Input: part model. Units: mm. Frame: model coordinates. Round coordinates to 2 decimals unless told otherwise and drop trailing zeros. Write each loop counter-clockwise with the first axis right and the second up, starting at its lowest first coordinate (ties: lowest second). Pieces come first, ordered by that corner, then holes. Notation, with made-up numbers: (11, 0.25) - (32, 0.25) arc R14 cw to (32, 9.25) - close; hole circle Ø8 at (-26.5, -7). An arc over 180 degrees is marked (long way). Use one line per item in the form item = value.
```python
from build123d import *

# Parameters (mm, degrees)
CHAMFER1_SIZE      = 0.25
CUT_EXTRUDE1_DEPTH = 0.5
FILLET7_R          = 0.5


with BuildPart() as part:
    # Sketch1 → Revolve1 (revolve)
    with BuildSketch(Plane(origin=(0, 0, 0), x_dir=(0, 0, -1), z_dir=(1, 0, 0))):
        Polygon((9.5, 0), (9.5, 1.5), (1.5, 1.5), (1.5, 2.5), (0, 2.5), (0, 0), align=None)
    revolve(axis=Axis((0, 0, 0), (0, 0, -1)))

    # Chamfer1
    chamfer1_edges = [part.edges().sort_by_distance(p)[0] for p in [
        (0, -1.5, -9.5),
    ]]
    chamfer(chamfer1_edges, length=CHAMFER1_SIZE)

    # Sketch2 → Cut-Extrude1 (cut)
    with BuildSketch(Plane.XY):
        with BuildLine():
            Line((-0.15, 2.495495943), (-0.15, 0.15))
            Line((-0.15, 0.15), (-2.495495943, 0.15))
            ThreePointArc((-2.495495943, 0.15), (-2.5, 0), (-2.495495943, -0.15))
            Line((-2.495495943, -0.15), (-0.15, -0.15))
            Line((-0.15, -0.15), (-0.15, -2.495495943))
            ThreePointArc((-0.15, -2.495495943), (0, -2.5), (0.15, -2.495495943))
            Line((0.15, -2.495495943), (0.15, -0.15))
            Line((0.15, -0.15), (2.495495943, -0.15))
            ThreePointArc((2.495495943, -0.15), (2.5, 0), (2.495495943, 0.15))
            Line((2.495495943, 0.15), (0.15, 0.15))
            Line((0.15, 0.15), (0.15, 2.495495943))
            ThreePointArc((0.15, 2.495495943), (0, 2.5), (-0.15, 2.495495943))
        make_face()
    extrude(amount=-CUT_EXTRUDE1_DEPTH, mode=Mode.SUBTRACT)

    # Fillet7
    fillet7_edges = [part.edges().sort_by_distance(p)[0] for p in [
        (-1.767766953, -1.767766953, 0),
        (1.767766953, -1.767766953, 0),
        (1.767766953, 1.767766953, 0),
        (-1.767766953, 1.767766953, 0),
    ]]
    fillet(fillet7_edges, radius=FILLET7_R)


solid = part.part
```
(1) Cut plane C-C on z = -2. Output: boundary loops of the cut face in (x, y).
Derived:
outline = circle Ø3 at (0, 0)
(2) Draft query along X for faces 1 (the face through (0, 0, -0.5)), 2 (the face through (0.07, -1.5, -5.32)), 3 (the face through (0, -2, -1.5)). Return one class per face: released by +X, released by -X, zero draft, split by the parting line, or undercut.
Derived:
face_1 = undercut
face_2 = split by the parting line
face_3 = zero draft
(3) First-contact query: pin 1 Ø2.5 at (x, y) = (1, -1) entering from -Z; pin 2 Ø1.5 at (x, z) = (1.5, -6) entering from -Y. Flat tips, straight axial feed; report the tip coordinate or a pass-through.
Derived:
pin_1 = -9.5
pin_2 = -1.3
(4) Material intervals for L1, parallel to Z at x = 0.8, y = 1.55; L2, parallel to Y at x = 1.1, z = -3.5; L3, parallel to X at y = 1.05, z = -3.75, sorted ascending.
Derived:
L1 = -1.5 to 0
L2 = -1.02 to 1.02
L3 = -1.07 to 1.07
(5) Cut plane A-A on x = 0. Output: boundary loops of the cut face in (y, z), then the cut area to 3 significant figures.
Derived:
outline = (-2.5, -1.5) - (-1.5, -1.5) - (-1.5, -9.25) - (-1.25, -9.5) - (1.25, -9.5) - (1.5, -9.25) - (1.5, -1.5) - (2.5, -1.5) - (2.5, -0.5) - (-2.5, -0.5) - close
area = 28.9 mm^2
